Could you check a few things on this model? Use its own coordinates, in mm. Round coordinates to 2 decimals unless told otherwise and drop trailing zeros. Write each loop counter-clockwise with the first axis right and the second up, starting at its lowest first coordinate (ties: lowest second). Pieces come first, ordered by that corner, then holes. Notation, with made-up numbers: (33.5, 65) -> (51.5, 65) arc R21 ccw to (51.5, 71) -> close; hole circle Ø7 at (64, -34.75). An arc over 180 degrees is marked (long way). Answer in a Markdown table with one row per item.
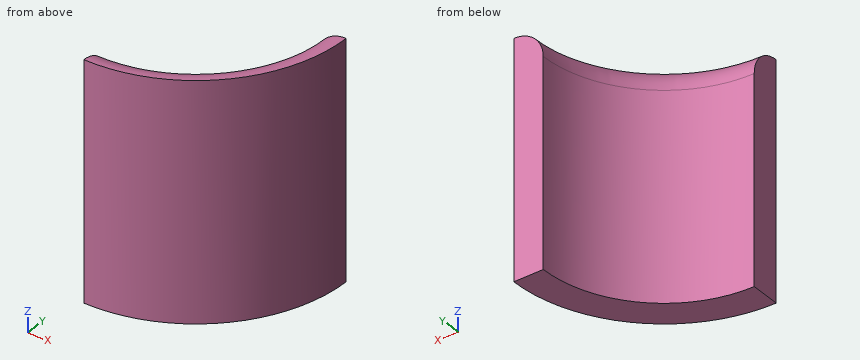
from build123d import *

# Parameters (mm, degrees)
SKETCH_1_R          = 510
SKETCH_1_R_2        = 410
EXTRUDE_1_DEPTH     = 800
FILLET_1_R          = 100
CUT_EXTRUDE_2_DEPTH = 800


with BuildPart() as part:
    # 草图1 → 凸台-拉伸1 (new body)
    with BuildSketch(Plane.XY):
        Circle(SKETCH_1_R)
        Circle(SKETCH_1_R_2, mode=Mode.SUBTRACT)
    extrude(amount=EXTRUDE_1_DEPTH)

    # 圆角1
    fillet_1_edges = [part.edges().sort_by_distance(p)[0] for p in [
        (-410, 0, 800),
    ]]
    fillet(fillet_1_edges, radius=FILLET_1_R - 0.0001)  # a hair under: the kernel refuses the full size

    # 草图2 → 切除-拉伸2 (cut)
    with BuildSketch(Plane.XY):
        Polygon((0, 764.183670641), (-976.361078065, 764.183670641), (-976.361078065, 0), (-976.361078065, -891.83511901), (0, -891.83511901), (0, 0), (1031.561704387, 0), (1031.561704387, 764.183670641), align=None)
    extrude(amount=CUT_EXTRUDE_2_DEPTH, mode=Mode.SUBTRACT)


solid = part.part
1) Imagine slicing it at A-A, the plane z = 118.5. Please give me the cut outline in (x, y), plus the area to 3 significant figures.
Findings:
| item | result |
|---|---|
| outline | (0, -510) arc R510 ccw to (510, 0) -> (410, 0) arc R410 cw to (0, -410) -> close |
| area | 72,300 mm^2 |
2) For pin 1 (2 mm diameter, centred on y = -308.5, z = 382.5, fed in from -X); pin 2 (12 mm diameter, centred on x = 251.5, z = 170.5, fed in from -Y); pin 3 (10 mm diameter, centred on y = -122.5, z = 662.5, fed in from +X), each with a flat end and sliding along its axis, tell me the tip position at first contact or that it passes through.
Findings:
| item | result |
|---|---|
| pin 1 | stops at x = 268.9 |
| pin 2 | stops at y = -447.02 |
| pin 3 | stops at x = 496.28 |
3) Please list where these lines run through material, in increasing order: line 1 (X direction, y = -432, z = 658.5); line 2 (Y direction, x = 245.5, z = 561); line 3 (Y direction, x = 132, z = 206.5).
Findings:
| item | result |
|---|---|
| line 1 | x = 0 to 271.06 |
| line 2 | y = -447.02 to -328.37 |
| line 3 | y = -492.62 to -388.17 |
